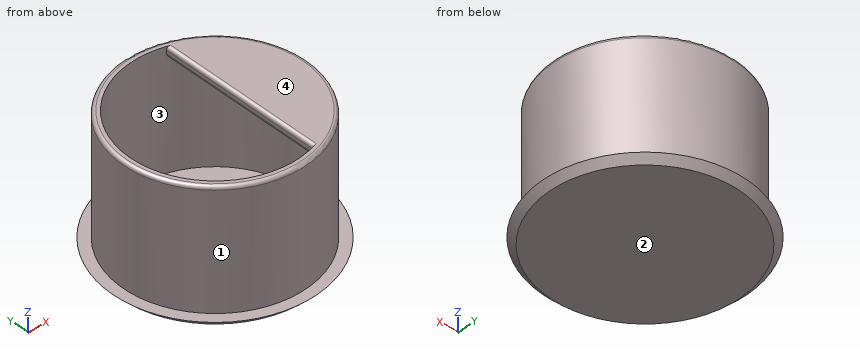
```python
from build123d import *

# Parameters (mm, degrees)
F0_R     = 26.875
F0_R_2   = 24.875
F1_DEPTH = 37
F0_R_3   = 30
F2_DEPTH = 2
F4_DEPTH = 3
F5_R     = 1
F6_SIZE  = 1.99999


# Not quite as in the source:
# - a fillet or chamfer is up to 0.001 mm smaller than in the source, because OpenCascade refuses the exact size


with BuildPart() as f1:
    # F0 (on Top) → F1 (new body)
    with BuildSketch(Plane.XY):
        Circle(F0_R)
        Circle(F0_R_2, mode=Mode.SUBTRACT)
    extrude(amount=F1_DEPTH)

    # F0 (on Top) → F2 (join)
    with BuildSketch(Plane.XY):
        Circle(F0_R_3)
        Circle(F0_R, mode=Mode.SUBTRACT)
        Circle(F0_R_2)
    extrude(amount=F2_DEPTH)

    # F3 (on face) → F4 (join)
    with BuildSketch(Plane.XY.offset(37)):
        with BuildLine():
            ThreePointArc((7.3629554948, -23.7603137896), (20.0239749167, -14.7582537427), (24.875, 0))
            ThreePointArc((24.875, 0), (20.0239749167, 14.7582537427), (7.3629554948, 23.7603137896))
            Line((7.3629554948, 23.7603137896), (7.3629554948, -23.7603137896))
        make_face()
    extrude(amount=-F4_DEPTH)

    # F5
    f5_edges = [f1.edges().sort_by_distance(p)[0] for p in [
        (7.362955, 0, 34),
        (7.362955, 0, 37),
        (-26.875, 0, 37),
    ]]
    fillet(f5_edges, radius=F5_R)

    # F6 (size 2 in the source; OpenCascade refuses exactly that, so slightly less here)
    f6_edges = [f1.edges().sort_by_distance(p)[0] for p in [
        (-30, 0, 0),
    ]]
    chamfer(f6_edges, length=F6_SIZE)


solid = f1.part
```
Input: part model. Units: mm. Frame: model coordinates. Face numbers are marked on the shaded views. Round coordinates to 2 decimals unless told otherwise and drop trailing zeros. Loops run counter-clockwise (first coordinate to the right, second up) from the corner with the lowest first, then second, coordinate; pieces in that order, holes last. Notation, with made-up numbers: (60.25, -9.75) -> (76.25, -9.75) arc R27 ccw to (76.25, 8.25) -> close; hole circle Ø8 at (53.25, 69.5). An arc over 180 degrees is marked (long way). One line per item, written item: value.
(1) Section C-C (z = 11.5). Return the cut outline in (x, y) (3 decimals), plus the area to 3 significant figures.
Geometry check:
outline: circle Ø53.75 at (0, 0); hole circle Ø49.75 at (0, 0)
area: 325 mm2
(2) Material intervals for line 1 (Z direction, x = 19.5, y = -7.5); line 2 (Y direction, x = 0, z = 9) (3 decimals); line 3 (Y direction, x = 19, z = 32), sorted ascending. Write a range as [from, to].
Geometry check:
line 1: [0, 2], [34, 37]
line 2: [-26.875, -24.875], [24.875, 26.875]
line 3: [-19.01, -16.06], [16.06, 19.01]
(3) Mould query, pull axis Z, two halves, no side actions, for the marked faces 1, 2, 3 and 4. Classes: pulls with the +Z half, pulls with the -Z half, needs draft (parallel to the pull), parting line crosses it, or undercut.
Geometry check:
face 1: needs draft
face 2: pulls with the -Z half
face 3: undercut
face 4: pulls with the +Z half
(4) Pin query (flat end, axial travel): pin 1 (4 mm diameter, centred on x = -22, y = 21.5, fed in from +Z); pin 2 (6 mm diameter, centred on y = 4, z = 8, fed in from +X); pin 3 (0.8 mm diameter, centred on y = 5.5, z = 35.5, fed in from -X). Return the tip coordinate at first contact, or that it passes through.
Geometry check:
pin 1: z = 2
pin 2: x = 26.86
pin 3: x = -26.39
